Drawing for the job (mm, zero at the part's lowest x, y, z). Round coordinates to 2 decimals unless told otherwise and drop trailing zeros. Write each loop counter-clockwise with the first axis right and the second up, starting at its lowest first coordinate (ties: lowest second). Pieces come first, ordered by that corner, then holes. Notation, with made-up numbers: (1.25, 66.5) -> (58.25, 66.5) arc R31 cw to (58.25, 100.5) -> close; hole circle Ø8 at (29.5, 69). An arc over 180 degrees is marked (long way). One line per question, with ' | ' between items.
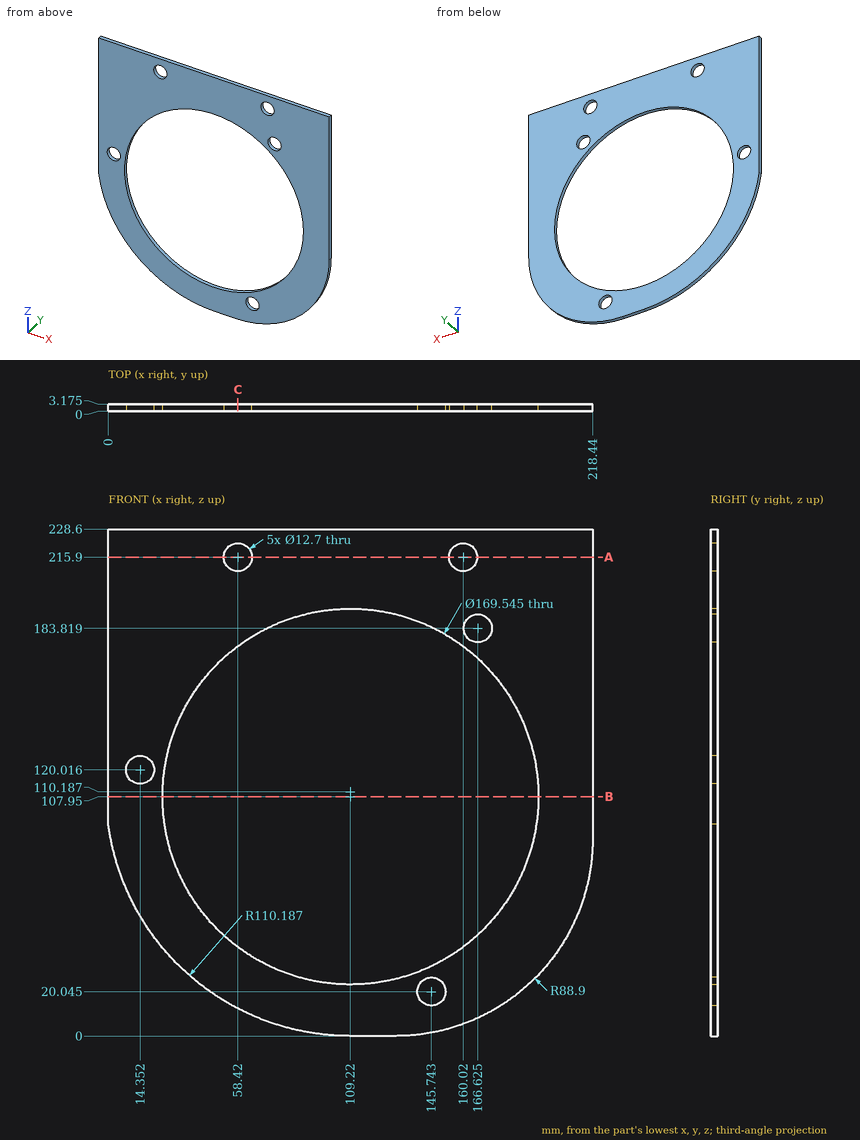
(1) Wall check: line 1 (X direction, y = 2.7, z = 216); line 2 (X direction, y = 2.4, z = 123) (1 decimal); line 3 (Z direction, x = 155.5, y = 2.4) (1 decimal). Give the ranges that are in metal, low to high. Write a range as from..to.
Calculated:
line 1: 0..52.07, 64.77..153.67, 166.37..218.44 | line 2: 0..8.7, 20..25.8, 192.6..218.4 | line 3: 3.9..36.9, 179..211.4, 220.4..228.6
(2) Slice it at B-B (z = 107.95). Write the cut outline in (x, y) (1 decimal), then the cut area to 3 significant figures.
Calculated:
outline: (0, 0) -> (24.4, 0) -> (24.4, 3.2) -> (0, 3.2) -> close; (194, 0) -> (218.4, 0) -> (218.4, 3.2) -> (194, 3.2) -> close | area: 155 mm2
(3) Drop a flat-ended pin along its axis: pin 1 (7.5 mm diameter, centred on x = 166.63, z = 183.82, fed in from -Y). Give the stop position or say it passes through.
Calculated:
pin 1: through
(4) Slice it at A-A (z = 215.9). Write the cut outline in (x, y) (1 decimal).
Calculated:
outline: (0, 0) -> (52.1, 0) -> (52.1, 3.2) -> (0, 3.2) -> close; (64.8, 0) -> (153.7, 0) -> (153.7, 3.2) -> (64.8, 3.2) -> close; (166.4, 0) -> (218.4, 0) -> (218.4, 3.2) -> (166.4, 3.2) -> close
(5) Slice it at C-C (x = 58.42). State how many separate pieces and enclosed holes the cut face has, then the cut area to 3 significant figures.
Calculated:
separate pieces: 3 | enclosed holes: 0 | area: 215 mm2
